Autodesk Inventor part; units mm, degrees
ref_plane "YZ Plane" through (0, 0, 0) normal (1, 0, 0) x (0, 1, 0)
ref_plane "XZ Plane" through (0, 0, 0) normal (0, 1, 0) x (-1, 0, 0)
ref_plane "XY Plane" through (0, 0, 0) normal (0, 0, 1) x (1, 0, 0)
sketch "Sketch1" plane through (0, 0, 0) normal (0, 0, 1) x (1, 0, 0)
  line L0 (3, 0) -> (97, 0)
  line L1 (100, 3) -> (100, 97)
  line L2 (97, 100) -> (3, 100)
  line L3 (0, 97) -> (0, 3)
  line L4 (4, 96) -> (96, 96) construction
  line L5 (96, 96) -> (96, 4) construction
  line L6 (96, 4) -> (4, 4) construction
  line L7 (4, 4) -> (4, 96) construction
  arc A0 (3, 100) -> (0, 97) centre (3, 97) ccw
  arc A1 (0, 3) -> (3, 0) centre (3, 3) ccw
  arc A2 (97, 0) -> (100, 3) centre (97, 3) ccw
  arc A3 (100, 97) -> (97, 100) centre (97, 97) ccw
  circle A4 centre (4, 96) radius 2
  circle A5 centre (4, 4) radius 2
  circle A6 centre (96, 4) radius 2
  circle A7 centre (96, 96) radius 2
  circle A8 centre (50, 50) radius 15
  circle A9 centre (50, 50) radius 10
  point P0 (0, 0)
  point P1 (100, 100)
  point P2 (100, 0)
  point P3 (0, 100)
  point P4 (50, 96)
  point P5 (4, 50)
  dimension "d0" = 100
  dimension "d1" = 100
  dimension "d2" = 4
  dimension "d3" = 3
  dimension "d4" = 4
  dimension "d5" = 20
  dimension "d6" = 30
extrude "Extrusion1" add sketch "Sketch1" against normal blind 3 contours A1 L3 A0 L2 A3 L1 A2 L0 | A8 | A9
extrude "Extrusion2" add sketch "Sketch1" along normal blind 15 contours A8
extrude "Extrusion3" add sketch "Sketch1" along normal blind 10 contours A9
chamfer "Chamfer1" distance 2 angle 45 1 edges at (40, 50, 15)
properties part number "CAMERA"
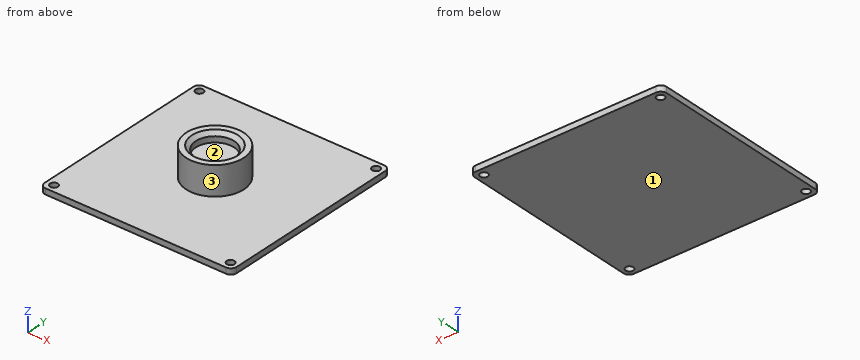
Geometry check sheet. Reference: the model listing, model coordinates, mm. Face numbers are marked on the shaded views. Give positions to 0.01 mm unless a question says otherwise; leave off trailing zeros. Order: outer loops, then holes, each group sorted by start corner. A loop starts at its lowest first (then second) coordinate and runs counter-clockwise, first axis right, second up.
1. Section check B-B, the plane y = 91.5. Enter the section's corners in (x, z).
2. Release check for a two-part mould opening along Y. For the marked faces 1, 2 and 3 record: pulls with the +Y half, pulls with the -Y half, needs draft (parallel to the pull), parting line crosses it, or undercut.
3. Section check C-C, the plane z = 3.75. Enter the section's corners in (x, y), and give its area (3 significant figures).
4. Thickness scan on L1, parallel to Y at x = 4, z = -1; L2, parallel to Z at x = 90, y = 19; L3, parallel to X at y = 39.5, z = 9.75. Record the ranges inside material, lowest first.
5. Section check A-A, the plane x = 50. Enter the section's corners in (y, z).
6. Gauge pin test, flat ends, axial feed: pin 1 Ø8 at (x, z) = (50, 12.5) entering from +Y; pin 2 Ø3 at (x, y) = (4, 4) entering from -Z; pin 3 Ø5 at (x, y) = (96, 96) entering from +Z; pin 4 Ø18 at (x, y) = (50, 50) entering from +Z. Record the tip position at first contact, or that the pin passes through.
Values follow:
1. outline: (0, -3) - (100, -3) - (100, 0) - (0, 0) - close
2. face 1: needs draft
2. face 2: undercut
2. face 3: parting line crosses it
3. outline: circle Ø30 at (50, 50)
3. area: 707 mm2
4. L1: y = 0 to 2, 6 to 94, 98 to 100
4. L2: z = -3 to 0
4. L3: x = 39.29 to 60.71
5. outline: (0, -3) - (100, -3) - (100, 0) - (65, 0) - (65, 15) - (62, 15) - (60, 13) - (60, 10) - (40, 10) - (40, 13) - (38, 15) - (35, 15) - (35, 0) - (0, 0) - close
6. pin 1: stops at y = 65
6. pin 2: passes through
6. pin 3: stops at z = 0
6. pin 4: stops at z = 10
